```python
from build123d import *

# Parameters (mm, degrees)
SKETCH045_R     = 1.05
PAD031_DEPTH    = 1
SKETCH046_W     = 6.3
SKETCH046_H     = 6.3
POCKET013_DEPTH = 1.001
SKETCH047_W     = 13
SKETCH047_H     = 9
POCKET014_DEPTH = 1.001
SKETCH049_W     = 1.5
SKETCH049_H     = 53
PAD032_DEPTH    = 1
FILLET001_R     = 0.5
FILLET002_R     = 0.5
FILLET003_R     = 0.5
SKETCH048_W     = 1.5
SKETCH048_H     = 6.181126
PAD033_DEPTH    = 1


with BuildPart() as part:
    # Sketch045 → Pad031 (new body)
    with BuildSketch(Plane.XY):
        with BuildLine():
            Line((-4, 71), (-4, 1))
            ThreePointArc((-4, 1), (-2.535534, -2.535534), (1, -4))
            Line((1, -4), (101, -4))
            ThreePointArc((101, -4), (104.535534, -2.535534), (106, 1))
            Line((106, 1), (106, 71))
            ThreePointArc((106, 71), (104.535534, 74.535534), (101, 76))
            Line((101, 76), (1, 76))
            ThreePointArc((1, 76), (-2.535534, 74.535534), (-4, 71))
        make_face()
        with Locations((1, 71)):
            Circle(SKETCH045_R, mode=Mode.SUBTRACT)
        with Locations((1, 1)):
            Circle(SKETCH045_R, mode=Mode.SUBTRACT)
        with Locations((101, 1)):
            Circle(SKETCH045_R, mode=Mode.SUBTRACT)
        with Locations((101, 71)):
            Circle(SKETCH045_R, mode=Mode.SUBTRACT)
    extrude(amount=PAD031_DEPTH)

    # Sketch046 (on Face14 of Pad031) → Pocket013 (cut, through all)
    with BuildSketch(Plane.XY.offset(1)):
        with Locations((89.27, 63.94)):
            Rectangle(SKETCH046_W, SKETCH046_H)
        with Locations((89.27, 51.24)):
            Rectangle(SKETCH046_W, SKETCH046_H)
        with Locations((89.27, 43.62)):
            Rectangle(SKETCH046_W, SKETCH046_H)
        with Locations((89.27, 30.92)):
            Rectangle(SKETCH046_W, SKETCH046_H)
        with Locations((89.27, 23.3)):
            Rectangle(SKETCH046_W, SKETCH046_H)
        with Locations((89.27, 10.6)):
            Rectangle(SKETCH046_W, SKETCH046_H)
        with Locations((15.6, 67.19)):
            Rectangle(SKETCH046_W, SKETCH046_H)
        with Locations((33.38, 67.19)):
            Rectangle(SKETCH046_W, SKETCH046_H)
        with Locations((48.62, 67.19)):
            Rectangle(SKETCH046_W, SKETCH046_H)
        with Locations((66.4, 67.19)):
            Rectangle(SKETCH046_W, SKETCH046_H)
    extrude(amount=-POCKET013_DEPTH, mode=Mode.SUBTRACT)

    # Sketch047 (on Face5 of Pocket013) → Pocket014 (cut, through all)
    with BuildSketch(Plane.XY.offset(1)):
        with Locations((14, 52.5)):
            Rectangle(SKETCH047_W, SKETCH047_H)
        with Locations((14, 39.166667)):
            Rectangle(SKETCH047_W, SKETCH047_H)
        with Locations((14, 25.833333)):
            Rectangle(SKETCH047_W, SKETCH047_H)
        with Locations((14, 12.5)):
            Rectangle(SKETCH047_W, SKETCH047_H)
        with Locations((33, 39.166667)):
            Rectangle(SKETCH047_W, SKETCH047_H)
        with Locations((33, 25.833333)):
            Rectangle(SKETCH047_W, SKETCH047_H)
        with Locations((33, 12.5)):
            Rectangle(SKETCH047_W, SKETCH047_H)
        with Locations((49, 39.166667)):
            Rectangle(SKETCH047_W, SKETCH047_H)
        with Locations((49, 25.833333)):
            Rectangle(SKETCH047_W, SKETCH047_H)
        with Locations((49, 12.5)):
            Rectangle(SKETCH047_W, SKETCH047_H)
        with Locations((66, 39.166667)):
            Rectangle(SKETCH047_W, SKETCH047_H)
        with Locations((66, 25.833333)):
            Rectangle(SKETCH047_W, SKETCH047_H)
        with Locations((66, 12.5)):
            Rectangle(SKETCH047_W, SKETCH047_H)
        with Locations((33, 52.5)):
            Rectangle(SKETCH047_W, SKETCH047_H)
        with Locations((49, 52.5)):
            Rectangle(SKETCH047_W, SKETCH047_H)
        with Locations((66, 52.5)):
            Rectangle(SKETCH047_W, SKETCH047_H)
    extrude(amount=-POCKET014_DEPTH, mode=Mode.SUBTRACT)

    # Sketch049 (on Face5 of Pocket014) → Pad032 (join)
    with BuildSketch(Plane.XY.offset(1)):
        with Locations((23.5, 32.5)):
            Rectangle(SKETCH049_W, SKETCH049_H)
        with Locations((41, 32.5)):
            Rectangle(SKETCH049_W, SKETCH049_H)
        with Locations((57.5, 32.5)):
            Rectangle(SKETCH049_W, SKETCH049_H)
        with Locations((74.5, 32.5)):
            Rectangle(SKETCH049_W, SKETCH049_H)
    extrude(amount=PAD032_DEPTH)

    # Fillet001
    fillet001_edges = [part.edges().sort_by_distance(p)[0] for p in [
        (24.25, 32.5, 2),
        (23.5, 6, 2),
        (22.75, 32.5, 2),
        (23.5, 59, 2),
    ]]
    fillet(fillet001_edges, radius=FILLET001_R)

    # Fillet002
    fillet002_edges = [part.edges().sort_by_distance(p)[0] for p in [
        (41, 59, 2),
        (41.75, 32.5, 2),
        (41, 6, 2),
        (40.25, 32.5, 2),
    ]]
    fillet(fillet002_edges, radius=FILLET002_R)

    # Fillet003
    fillet003_edges = [part.edges().sort_by_distance(p)[0] for p in [
        (57.5, 59, 2),
        (58.25, 32.5, 2),
        (57.5, 6, 2),
        (56.75, 32.5, 2),
        (74.5, 59, 2),
        (75.25, 32.5, 2),
        (74.5, 6, 2),
        (73.75, 32.5, 2),
    ]]
    fillet(fillet003_edges, radius=FILLET003_R)

    # Sketch048 (on Face5 of Pocket014) → Pad033 (join)
    with BuildSketch(Plane.XY.offset(1)):
        Polygon((94.197178, 10.6), (96.737139, 9.774717), (96.737139, 7.104044), (98.306921, 9.264664), (100.846882, 8.43938), (99.2771, 10.6), (100.846882, 12.76062), (98.306921, 11.935336), (96.737139, 14.095956), (96.737139, 11.425283), align=None)
        with Locations((97.873044, 30.92)):
            Rectangle(SKETCH048_W, SKETCH048_H)
        Polygon((97.123044, 26.390563), (98.623044, 26.390563), (98.623044, 24.05), (100.963607, 24.05), (100.963607, 22.55), (98.623044, 22.55), (98.623044, 20.209437), (97.123044, 20.209437), (97.123044, 22.55), (94.782481, 22.55), (94.782481, 24.05), (97.123044, 24.05), align=None)
        Polygon((94.244044, 43.62), (97.873044, 41.524796), (97.873044, 45.715204), align=None)
        Polygon((101.502044, 51.24), (97.873044, 53.335204), (97.873044, 49.144796), align=None)
        Polygon((97.287938, 67.569), (95.192734, 63.94), (99.383142, 63.94), align=None)
    extrude(amount=PAD033_DEPTH)


with BuildPart() as part_1:
    # Body008 placement: moved
    add(part.part.moved(Location((0, 0, 8))))


solid = part_1.part
```
Verification items for the finished model (mm, model axes). A direction names the side the tool comes from. Round coordinates to 2 decimals unless told otherwise and drop trailing zeros. Write each loop counter-clockwise with the first axis right and the second up, starting at its lowest first coordinate (ties: lowest second). Pieces come first, ordered by that corner, then holes.
1. Access from +Z, -Z, +X, -X, +Y, -Y to the whole of each face (thin tool, end or side, straight path). Record for faces 1 (the flat face through (99.713, 52.273, 9.493)), 2 (the cylindrical face through (-2.5, 74.57, 8.49)), 3 (the flat face through (96.255, 65.78, 9.493)), 4 (the flat face through (96.08, 44.68, 9.49)).
2. Scan lines: L1, parallel to Y at x = 1, z = 8.85; L2, parallel to X at y = 54, z = 8.1; L3, parallel to X at y = 19, z = 9.5. Record each from-to range of solid material in increasing order.
3. Section check A-A on x = 14. Enter the section's corners in (y, z), plus the area to 3 significant figures.
4. Draft check along Y on faces 5 (the cylindrical face through (104.5, -2.57, 8.49)), 6 (the flat face through (96, 44, 10)), 7 (the flat face through (99.7, 50.2, 9.5)). Enter one of: +Y half, -Y half, draft (parallel to the pull), parting line (faces both ways), or undercut.
5. Gauge pin test, flat ends, axial feed: P1, Ø6, axis at x = 62, y = 36.5, coming from the +Z side; P2, Ø10, axis at x = 52, y = 46.5, coming from the +Z side; P3, Ø0.8, axis at x = 96, z = 9.5, coming from the +Y side. Record the tip position at first contact, or that the pin passes through.
6. Section check B-B on y = 62. Enter the section's corners in (x, z), plus the area to 3 significant figures.
7. Section check C-C on z = 8.4. State how many separate pieces and enclosed holes the cut face has, plus the area to 3 significant figures.
8. Section check D-D on x = 81. Enter the section's corners in (y, z), plus the area to 3 significant figures.
Answer:
1. face 1: +Z, +X
1. face 2: +Z, -Z, -X, +Y
1. face 3: +Z, -X, +Y
1. face 4: +Z
2. L1: y = -4 to -0.05, 2.05 to 69.95, 72.05 to 76
2. L2: x = -4 to 7.5, 20.5 to 26.5, 39.5 to 42.5, 55.5 to 59.5, 72.5 to 86.12, 92.42 to 106
2. L3: x = 22.75 to 24.25, 40.25 to 41.75, 56.75 to 58.25, 73.75 to 75.25
3. outline: (-4, 8) - (8, 8) - (8, 9) - (-4, 9) - close; (17, 8) - (21.33, 8) - (21.33, 9) - (17, 9) - close; (30.33, 8) - (34.67, 8) - (34.67, 9) - (30.33, 9) - close; (43.67, 8) - (48, 8) - (48, 9) - (43.67, 9) - close; (57, 8) - (64.04, 8) - (64.04, 9) - (57, 9) - close; (70.34, 8) - (76, 8) - (76, 9) - (70.34, 9) - close
3. area: 37.7 mm2
4. face 5: -Y half
4. face 6: draft
4. face 7: undercut
5. P1: stops at z = 9
5. P2: stops at z = 9.93
5. P3: stops at y = 66.03
6. outline: (-4, 8) - (86.12, 8) - (86.12, 9) - (-4, 9) - close; (92.42, 8) - (106, 8) - (106, 9) - (92.42, 9) - close
6. area: 104 mm2
7. separate pieces: 1
7. enclosed holes: 30
7. area: 6,500 mm2
8. outline: (-4, 8) - (76, 8) - (76, 9) - (-4, 9) - close
8. area: 80.0 mm2
